Can you work these out from the drawing? Everything is in mm from the part's minimum corner. Give positions to 0.01 mm unless a question says otherwise; leave off trailing zeros. Loops run counter-clockwise (first coordinate to the right, second up) from the corner with the lowest first, then second, coordinate; pieces in that order, holes last. Notation, with made-up numbers: (6, -14.5) -> (65, -14.5) arc R14 ccw to (65, -1.5) -> close; hole circle Ø6 at (56, 6). An arc over 180 degrees is marked (long way). Write item = value, one per line. Start each with the question number.
1) If we mould it in two halves opening along Y, with no side actions, what happens to the marked faces 1, 2 and 3? For each: +Y half, -Y half, draft (parallel to the pull), parting line (faces both ways), or undercut.
2) I want a section at B-B (x = 3.5). List the corners of the cut face in (y, z) for me (1 decimal), and give its area (3 significant figures).
3) I want a section at A-A (y = 33.02). List the corners of the cut face in (x, z) for me (1 decimal).
4) I want a section at C-C (z = 2.4). List the corners of the cut face in (x, y) for me (1 decimal), and give its area (3 significant figures).
5) I need wall thicknesses on probe 1 along Y at (x, z) = (5, 2.35); probe 2 along Y at (x, z) = (3.75, 2.1); probe 3 along X at (y, z) = (11.5, 2.8). Which ranges of each line are inside material? Lowest first, please. Write a range as from..to.
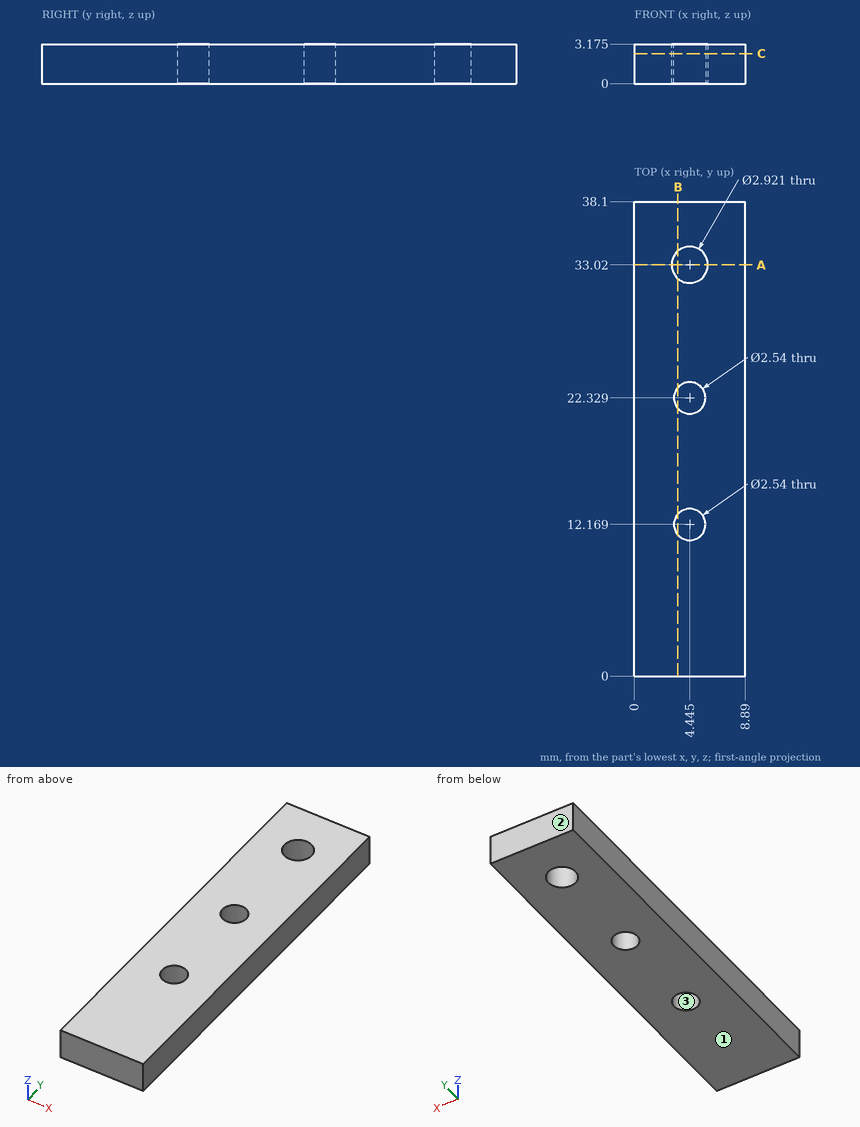
Answer list:
q1.face_1 = draft
q1.face_2 = +Y half
q1.face_3 = undercut
q2.outline = (0, 0) -> (11.3, 0) -> (11.3, 3.2) -> (0, 3.2) -> close; (13, 0) -> (21.5, 0) -> (21.5, 3.2) -> (13, 3.2) -> close; (23.2, 0) -> (31.9, 0) -> (31.9, 3.2) -> (23.2, 3.2) -> close; (34.1, 0) -> (38.1, 0) -> (38.1, 3.2) -> (34.1, 3.2) -> close
q2.area = 103 mm^2
q3.outline = (0, 0) -> (3, 0) -> (3, 3.2) -> (0, 3.2) -> close; (5.9, 0) -> (8.9, 0) -> (8.9, 3.2) -> (5.9, 3.2) -> close
q4.outline = (0, 0) -> (8.9, 0) -> (8.9, 38.1) -> (0, 38.1) -> close; hole circle Ø2.9 at (4.4, 33); hole circle Ø2.5 at (4.4, 12.2); hole circle Ø2.5 at (4.4, 22.3)
q4.area = 322 mm^2
q5.probe_1 = 0..11.03, 13.31..21.19, 23.47..31.67, 34.37..38.1
q5.probe_2 = 0..11.11, 13.23..21.27, 23.39..31.74, 34.3..38.1
q5.probe_3 = 0..3.37, 5.52..8.89
